from build123d import *

# Parameters (mm, degrees)
F1_DEPTH = 25.4
F2_W     = 5.2324
F2_H     = 2.9972
F3_DEPTH = 21.21


with BuildPart() as f1:
    # F0 (on Front) → F1 (new body)
    with BuildSketch(Plane.XZ):
        Polygon((-7.8359, 3.4925), (-7.8359, 0), (7.8359, 0), (7.8359, 3.4925), (10.6045, 6.2611), (10.6045, 6.7945), (8.0772, 9.3218), (-8.0772, 9.3218), (-10.6045, 6.7945), (-10.6045, 6.2611), align=None)
    extrude(amount=F1_DEPTH)

    # F2 (on face) → F3 (cut, through all)
    with BuildSketch(Plane.YZ.offset(10.6045)):
        with Locations((2.6162, 7.8232)):
            Rectangle(F2_W, F2_H)
        with Locations((-7.3914, 7.8232)):
            Rectangle(F2_W, F2_H)
        with Locations((-17.399, 7.8232)):
            Rectangle(F2_W, F2_H)
        with Locations((-27.4066, 7.8232)):
            Rectangle(F2_W, F2_H)
    extrude(amount=-F3_DEPTH, mode=Mode.SUBTRACT)


solid = f1.part
Source: CAD feature listing. Evaluate the final solid. Frame: model axes, mm. A direction names the side the tool comes from. Round coordinates to 2 decimals unless told otherwise and drop trailing zeros. Loops run counter-clockwise (first coordinate to the right, second up) from the corner with the lowest first, then second, coordinate; pieces in that order, holes last.
Q1. Ray query, line 1 (Y direction, x = -6.25, z = 6.5); line 2 (X direction, y = -10.5, z = 2.5); line 3 (Z direction, x = -2, y = -6.5). Return the intervals inside material, ascending.
Q2. Mould query, pull axis Y, two halves, no side actions, for faces 1 (the face through (0, 0, 5)), 2 (the face through (9.4, -12.4, 8)), 3 (the face through (0, -20.015, 8)). Classes: pulls with the +Y half, pulls with the -Y half, needs draft (parallel to the pull), parting line crosses it, or undercut.
Q3. First-contact query: P1, Ø1, axis at y = -18.5, z = 2, coming from the -X side; P2, Ø2.5, axis at x = 1.5, z = 8.5, coming from the -Y side; P3, Ø4, axis at y = -7, z = 2, coming from the +X side. Flat tips, straight axial feed; report the tip coordinate or a pass-through.
Q4. Section C-C, the plane z = 2. Return loops of the section in (x, y), plus the area to 3 significant figures.
Q5. Section D-D, the plane y = -23.5. Return loops of the section in (x, z), plus the area to 3 significant figures.
Q6. Access query for faces 4 (the face through (7.836, -13, 2)), 5 (the face through (-7.836, -13, 2)), 6 (the face through (0, -24.79, 8)), 7 (the face through (0, -17, 6.325)). Directions: +Z, -Z, +X, -X, +Y, -Y. A direction counts if a zero-diameter tool reaches every point of the face in a straight line with its end or side. Return the directions, or none.
Q7. Section B-B, the plane x = 2.5. Return loops of the section in (y, z), plus the area to 3 significant figures.
Q8. Section A-A, the plane y = -5.25. Return loops of the section in (x, z).
Solutions:
1. line 1: y = -24.79 to -20.02, -14.78 to -10.01, -4.78 to 0
1. line 2: x = -7.84 to 7.84
1. line 3: z = 0 to 6.32
2. face 1: pulls with the +Y half
2. face 2: needs draft
2. face 3: undercut
3. P1: stops at x = -7.84
3. P2: stops at y = -24.79
3. P3: stops at x = 8.34
4. outline: (-7.84, -25.4) - (7.84, -25.4) - (7.84, 0) - (-7.84, 0) - close
4. area: 398 mm2
5. outline: (-10.6, 6.26) - (-7.84, 3.49) - (-7.84, 0) - (7.84, 0) - (7.84, 3.49) - (10.6, 6.26) - (10.6, 6.79) - (8.08, 9.32) - (-8.08, 9.32) - (-10.6, 6.79) - close
5. area: 164 mm2
6. face 4: -Z, +X, +Y, -Y
6. face 5: -Z, -X, +Y, -Y
6. face 6: +Z, +X, -X, -Y
6. face 7: +Z, +X, -X
7. outline: (-25.4, 0) - (0, 0) - (0, 9.32) - (-4.78, 9.32) - (-4.78, 6.32) - (-10.01, 6.32) - (-10.01, 9.32) - (-14.78, 9.32) - (-14.78, 6.32) - (-20.02, 6.32) - (-20.02, 9.32) - (-24.79, 9.32) - (-24.79, 6.32) - (-25.4, 6.32) - close
7. area: 204 mm2
8. outline: (-10.6, 6.26) - (-7.84, 3.49) - (-7.84, 0) - (7.84, 0) - (7.84, 3.49) - (10.6, 6.26) - (10.6, 6.32) - (-10.6, 6.32) - close
